```python
from build123d import *

# Parameters (mm, degrees)
F1_R    = 0.762
F2_R    = 2.54
F7_R    = 0.254
F3_SIZE = 0.508
F4_R    = 0.254
F5_SIZE = 1.27


with BuildPart() as f6:
    # F0 (on Front) → F6 (revolve)
    with BuildSketch(Plane.XZ):
        Polygon((-27.69616, -0.77978), (-27.69616, -3.81), (-21.92782, -3.81), (-21.92782, -1.905), (-19.15414, -1.905), (-19.15414, 7.62), (-24.384, 7.62), (-24.384, 2.53238), align=None)
    revolve(axis=Axis((0, 0, 5.998353), (0, 0, -1)))

    # F1
    f1_edges = [f6.edges().sort_by_distance(p)[0] for p in [
        (27.69616, 0, -0.77978),
    ]]
    fillet(f1_edges, radius=F1_R)

    # F2
    f2_edges = [f6.edges().sort_by_distance(p)[0] for p in [
        (24.384, 0, 2.53238),
    ]]
    fillet(f2_edges, radius=F2_R)

    # F7
    f7_edges = [f6.edges().sort_by_distance(p)[0] for p in [
        (27.69616, 0, -3.81),
    ]]
    fillet(f7_edges, radius=F7_R)

    # F3
    f3_edges = [f6.edges().sort_by_distance(p)[0] for p in [
        (21.92782, 0, -3.81),
        (19.15414, 0, -1.905),
    ]]
    chamfer(f3_edges, length=F3_SIZE)

    # F4
    f4_edges = [f6.edges().sort_by_distance(p)[0] for p in [
        (21.92782, 0, -1.905),
    ]]
    fillet(f4_edges, radius=F4_R)

    # F5
    f5_edges = [f6.edges().sort_by_distance(p)[0] for p in [
        (24.384, 0, 7.62),
    ]]
    chamfer(f5_edges, length=F5_SIZE)


solid = f6.part
```
Source: CAD feature listing. Evaluate the final solid. Frame: model axes, mm. A direction names the side the tool comes from. Give positions to 0.01 mm unless a question says otherwise; leave off trailing zeros. Loops run counter-clockwise (first coordinate to the right, second up) from the corner with the lowest first, then second, coordinate; pieces in that order, holes last. Notation, with made-up numbers: M -21.5,-1 L 1.5,-1 A18 cw 1.5,7 Z; hole C -19,-10.5 d10. An arc over 180 degrees is marked long. Put each result on its own line as item: value.
Q1. Section A-A (z = 4.75). Return the cut outline in (x, y).
Response values:
outline: C 0,0 d48.77; hole C 0,0 d38.31
Q2. Line query: probe 1 along Y at (x, z) = (0, -2.5); probe 2 along Y at (x, z) = (0, 4.25); probe 3 along X at (y, z) = (18.5, -3.25). Output: solid intervals per line, ascending. Write a range as [from, to].
Response values:
probe 1: y = [-27.7, -21.93], [21.93, 27.7]
probe 2: y = [-24.38, -19.15], [19.15, 24.38]
probe 3: x = [-20.61, -11.77], [11.77, 20.61]
Q3. Mould query, pull axis X, two halves, no side actions, for faces 1 (the cylindrical face through (20.41, 18.72, -2.34)), 2 (the flat face through (-14, 14, 7.62)), 3 (the cylindrical face through (17.401, -13.343, -2.722)), 4 (the flat face through (4.9, -19.2, -1.905)). Classes: released by +X, released by -X, zero draft, split by the parting line, or undercut.
Response values:
face 1: split by the parting line
face 2: zero draft
face 3: undercut
face 4: undercut
Q4. Pin query (flat end, axial travel): P1, Ø6, axis at y = -14.5, z = 4, coming from the -X side; P2, Ø10, axis at x = 14, y = 3.5, coming from the -Z side; P3, Ø6, axis at x = 10.5, z = -1, coming from the +Y side. Return the tip coordinate at first contact, or that it passes through.
Response values:
P1: stops at x = -21.96
P2: stops at z = -1.67
P3: stops at y = 26.66
Q5. Reachability of faces 5 (the cylindrical face through (3.174, 24.177, 4.948)), 6 (the cylindrical face through (14.117, 12.945, 3.175)) from +Z, -Z, +X, -X, +Y, -Y: full face, straight path, thin tool, end or side. Return the list, or none.
Response values:
face 5: +Z
face 6: +Z, -Z
